```python
from build123d import *

# Parameters (mm, degrees)
SKETCH1_R           = 7
BOSS_EXTRUDE1_DEPTH = 3
SKETCH2_W           = 4
SKETCH2_H           = 7
SKETCH2_W_2         = 2
SKETCH2_H_2         = 5
BOSS_EXTRUDE2_DEPTH = 5
FILLET1_R           = 2


with BuildPart() as part:
    # Sketch1 → Boss-Extrude1 (new body)
    with BuildSketch(Plane(origin=(0, 0, 0), x_dir=(1, 0, 0), z_dir=(0, 1, 0))):
        Circle(SKETCH1_R)
    extrude(amount=BOSS_EXTRUDE1_DEPTH)

    # Sketch2 → Boss-Extrude2 (add)
    with BuildSketch(Plane(origin=(0, 3, 0), x_dir=(1, 0, 0), z_dir=(0, 1, 0))):
        Rectangle(SKETCH2_W, SKETCH2_H)
        Rectangle(SKETCH2_W_2, SKETCH2_H_2, mode=Mode.SUBTRACT)
    extrude(amount=BOSS_EXTRUDE2_DEPTH)

    # Fillet1
    fillet1_edges = [part.edges().sort_by_distance(p)[0] for p in [
        (-2, 3, 0),
        (0, 3, -3.5),
        (2, 3, 0),
        (0, 3, 3.5),
    ]]
    fillet(fillet1_edges, radius=FILLET1_R)


solid = part.part
```
Input: part model. Units: mm. Frame: model coordinates. A direction names the side the tool comes from. Coordinates: 2 decimals unless noted, no trailing zeros. Loops run counter-clockwise (first coordinate to the right, second up) from the corner with the lowest first, then second, coordinate; pieces in that order, holes last. Notation, with made-up numbers: M 37,30.5 L 74,30.5 A19 cw 74,54.5 Z; hole C -18,-32.75 d2. An arc over 180 degrees is marked long. Use a Markdown table: item, result. Add a question column.
1) Draft query along X for faces 1 (the flat face through (-1, 5, 0)), 2 (the flat face through (0, 6, -3.5)), 3 (the flat face through (2, 6, 0)). Return one class per face: +X half, -X half, draft (parallel to the pull), parting line (faces both ways), or undercut.
2) Line query: L1, parallel to X at y = 6.75, z = 1.75; L2, parallel to Z at x = -1.5, y = 6.75; L3, parallel to Y at x = 0.75, z = 1. Output: solid intervals per line, ascending. Write a range as from..to.
3) Pin query (flat end, axial travel): P1, Ø0.6, axis at x = -0.5, z = 1, coming from the +Y side; P2, Ø2.5, axis at y = 6.5, z = 1.5, coming from the +X side; P3, Ø3.5, axis at x = -0.5, y = 7, coming from the +Z side. Return the tip coordinate at first contact, or that it passes through.
4) Section C-C, the plane x = 0. Return the cut outline in (y, z).
5) Section B-B, the plane y = 4.25. Return the cut outline in (x, z), plus the area to 3 significant figures.
6) Section A-A, the plane z = 0. Return the cut outline in (x, y), plus the area to 3 significant figures.
7) Section D-D, the plane y = 2.75. Return the cut outline in (x, z), plus the area to 3 significant figures.
8) Set-up query: faces 4 (the flat face through (0, 6, 3.5)), 5 (the flat face through (0, 0, 0)), 6 (the flat face through (0, 5, 2.5)), 7 (the flat face through (-2, 6, 0)). Return all of +Z, -Z, +X, -X, +Y, -Y with unobstructed straight access to the full face (end or side cutting, diameter ignored); none if empty.
Answer below:
| question | item | result |
|---|---|---|
| 1 | face 1 | undercut |
| 1 | face 2 | draft |
| 1 | face 3 | +X half |
| 2 | L1 | -2..-1, 1..2 |
| 2 | L2 | -3.5..3.5 |
| 2 | L3 | 0..3 |
| 3 | P1 | y = 3 |
| 3 | P2 | x = 2 |
| 3 | P3 | z = 3.5 |
| 4 | outline | M 0,-7 L 3,-7 L 3,-5.5 A2 cw 5,-3.5 L 8,-3.5 L 8,-2.5 L 3,-2.5 L 3,2.5 L 8,2.5 L 8,3.5 L 5,3.5 A2 cw 3,5.5 L 3,7 L 0,7 Z |
| 5 | outline | M -2.15,-3.65 L 2.15,-3.65 L 2.15,3.65 L -2.15,3.65 Z; hole M -1,-2.5 L 1,-2.5 L 1,2.5 L -1,2.5 Z |
| 5 | area | 21.3 mm2 |
| 6 | outline | M -7,0 L 7,0 L 7,3 L 4,3 A2 cw 2,5 L 2,8 L 1,8 L 1,3 L -1,3 L -1,8 L -2,8 L -2,5 A2 cw -4,3 L -7,3 Z |
| 6 | area | 53.7 mm2 |
| 7 | outline | C 0,0 d14 |
| 7 | area | 154 mm2 |
| 8 | face 4 | +Z, +X, -X, +Y |
| 8 | face 5 | +Z, -Z, +X, -X, -Y |
| 8 | face 6 | +Y |
| 8 | face 7 | +Z, -Z, -X, +Y |
